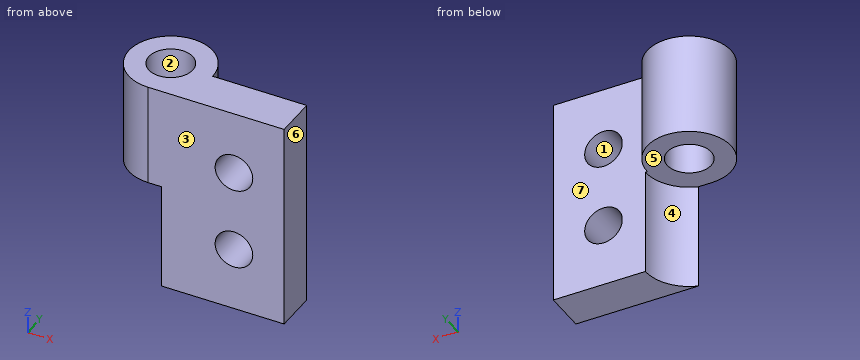
```python
from build123d import *

# Parameters (mm, degrees)
BOSS_EXTRUDE1_DEPTH = 25.4
SKETCH5_R           = 2.286
CUT_EXTRUDE3_DEPTH  = 12.954
SKETCH8_R           = 5.334
CUT_EXTRUDE5_DEPTH  = 12.954
SKETCH9_R           = 2.667
CUT_EXTRUDE6_DEPTH  = 12.7


with BuildPart() as part:
    # Sketch2 → Boss-Extrude1 (new body)
    with BuildSketch(Plane.XY):
        with BuildLine():
            Line((0, 0), (-16.51, 0))
            ThreePointArc((-16.51, 0), (-20.102102448, 8.672102448), (-11.43, 5.08))
            Line((-11.43, 5.08), (0, 5.08))
            Line((0, 5.08), (0, 0))
        make_face()
    extrude(amount=BOSS_EXTRUDE1_DEPTH)

    # Sketch5 → Cut-Extrude3 (cut)
    with BuildSketch(Plane(origin=(0, 5.08, 0), x_dir=(1, 0, 0), z_dir=(0, 1, 0))):
        with Locations((-6.096, -17.695333333)):
            Circle(SKETCH5_R)
        with Locations((-6.096, -7.704666667)):
            Circle(SKETCH5_R)
    extrude(amount=-CUT_EXTRUDE3_DEPTH, mode=Mode.SUBTRACT)

    # Sketch8 → Cut-Extrude5 (cut)
    with BuildSketch(Plane(origin=(0, 0, 0), x_dir=(-1, 0, 0), z_dir=(0, 0, -1))):
        with Locations((16.51, 5.08)):
            Circle(SKETCH8_R)
    extrude(amount=-CUT_EXTRUDE5_DEPTH, mode=Mode.SUBTRACT)

    # Sketch9 → Cut-Extrude6 (cut)
    with BuildSketch(Plane(origin=(0, 0, 12.954), x_dir=(-1, 0, 0), z_dir=(0, 0, -1))):
        with Locations((16.51, 5.08)):
            Circle(SKETCH9_R)
    extrude(amount=-CUT_EXTRUDE6_DEPTH, mode=Mode.SUBTRACT)


solid = part.part
```
Geometry check sheet. Reference: the model listing, model coordinates, mm. Face numbers are marked on the shaded views. A direction names the side the tool comes from. Give positions to 0.01 mm unless a question says otherwise; leave off trailing zeros. Order: outer loops, then holes, each group sorted by start corner. A loop starts at its lowest first (then second) coordinate and runs counter-clockwise, first axis right, second up. Notation, with made-up numbers: (85.25, 10) - (133.25, 10) arc R28 ccw to (133.25, 49) - close; hole circle Ø9 at (-36, 56). An arc over 180 degrees is marked (long way). Answer in a Markdown table with one row per item. Add a question column.
Q1. Cross-section at A-A, the plane y = 3.5. Enter the section's corners in (x, z).
Q2. Gauge pin test, flat ends, axial feed: pin 1 (5.5 mm diameter, centred on x = -6.1, z = 17.7, fed in from +Y); pin 2 (5 mm diameter, centred on x = -18, y = 3.5, fed in from -Z). Record the tip position at first contact, or that the pin passes through.
Q3. Cross-section at C-C, the plane y = 5.5. Enter the section's corners in (x, z), then the cut area to 3 significant figures.
Q4. Cross-section at D-D, the plane x = -6.5. Enter the section's corners in (y, z), then the cut area to 3 significant figures.
Q5. Tool access check on the marked faces 5, 6 and 7. Record the directions out of +Z, -Z, +X, -X, +Y, -Y that give a thin tool (end or side, any length) a straight path to the whole face; none if there is none.
Q6. Material ranges on probe 1 along Z at (x, y) = (-6, 3); probe 2 along Y at (x, z) = (-16.51, 17); probe 3 along X at (y, z) = (3.25, 16), recorded low to high. Write a range as from..to.
Q7. Cross-section at B-B, the plane z = 16.75. Enter the section's corners in (x, y), then the cut area to 3 significant figures.
Q8. Mould release check, pull along Y, two halves, no side actions. Record for the marked faces 1, 2, 3 and 4: pulls with the +Y half, pulls with the -Y half, needs draft (parallel to the pull), parting line crosses it, or undercut.
Check values:
| question | item | result |
|---|---|---|
| 1 | outline | (-21.34, 12.95) - (-18.66, 12.95) - (-18.66, 25.4) - (-21.34, 25.4) - close; (-14.36, 12.95) - (-11.42, 12.95) - (-11.42, 0) - (0, 0) - (0, 25.4) - (-14.36, 25.4) - close; hole circle Ø4.57 at (-6.1, 7.7); hole circle Ø4.57 at (-6.1, 17.7) |
| 2 | pin 1 | stops at y = 5.08 |
| 2 | pin 2 | stops at z = 12.95 |
| 3 | outline | (-21.57, 12.95) - (-19.14, 12.95) - (-19.14, 25.4) - (-21.57, 25.4) - close; (-13.88, 12.95) - (-11.45, 12.95) - (-11.45, 25.4) - (-13.88, 25.4) - close |
| 3 | area | 60.5 mm^2 |
| 4 | outline | (0, 0) - (5.08, 0) - (5.08, 5.45) - (0, 5.45) - close; (0, 9.95) - (5.08, 9.95) - (5.08, 15.45) - (0, 15.45) - close; (0, 19.95) - (5.08, 19.95) - (5.08, 25.4) - (0, 25.4) - close |
| 4 | area | 83.3 mm^2 |
| 5 | face 5 | -Z, -X, +Y |
| 5 | face 6 | +Z, -Z, +X, +Y, -Y |
| 5 | face 7 | +Z, -Z, +X, +Y |
| 6 | probe 1 | z = 0..5.42, 9.99..15.41, 19.98..25.4 |
| 6 | probe 2 | y = 0..2.41, 7.75..10.16 |
| 6 | probe 3 | x = -21.25..-18.45, -14.57..-7.63, -4.56..0 |
| 7 | outline | (-16.51, 0) - (-8.18, 0) - (-8.18, 5.08) - (-11.43, 5.08) arc R5.08 ccw (long way) to start; (-4.01, 0) - (0, 0) - (0, 5.08) - (-4.01, 5.08) - close; hole circle Ø5.33 at (-16.51, 5.08) |
| 7 | area | 101 mm^2 |
| 8 | face 1 | needs draft |
| 8 | face 2 | undercut |
| 8 | face 3 | pulls with the -Y half |
| 8 | face 4 | pulls with the +Y half |
